Read the model definition and answer for the solid it produces. Units are mm, in the model's axes. Coordinates: 2 decimals unless noted, no trailing zeros. Order: outer loops, then holes, each group sorted by start corner. A loop starts at its lowest first (then second) coordinate and runs counter-clockwise, first axis right, second up. Notation, with made-up numbers: M 30.25,82 L 41.25,82 A24 cw 41.25,105 Z; hole C 83.25,81 d10. An arc over 180 degrees is marked long. Use a Markdown table: item, result. Add a question column.
1) Each of these flat-tipped pins is pushed along its axis until it touches: pin 1 Ø1.3 at (y, z) = (-8.5, -1) entering from -X (3 decimals); pin 2 Ø3.5 at (y, z) = (4, 7.5) entering from -X (3 decimals); pin 3 Ø2 at (y, z) = (-4.76, 8.25) entering from -X. Where does it stop, or does it pass through?
2) Find section A-A on z = 0. Count the separate pieces of the cut face and the enclosed holes in it, plus the area to 3 significant figures.
3) Find section B-B on y = 0. Write down the section's boundary in (x, z) (3 decimals), plus the area to 3 significant figures.
4) Find section C-C on y = 49.5. Write down the section's boundary in (x, z) (3 decimals), plus the area to 3 significant figures.
5) Find the intervals of material crossed by probe 1 along Y at (x, z) = (-0.5, 0) (3 decimals); probe 2 along Y at (x, z) = (-1.25, 0) (3 decimals); probe 3 along Z at (x, y) = (1, -31) (3 decimals), in increasing order. Write a range as [from, to].
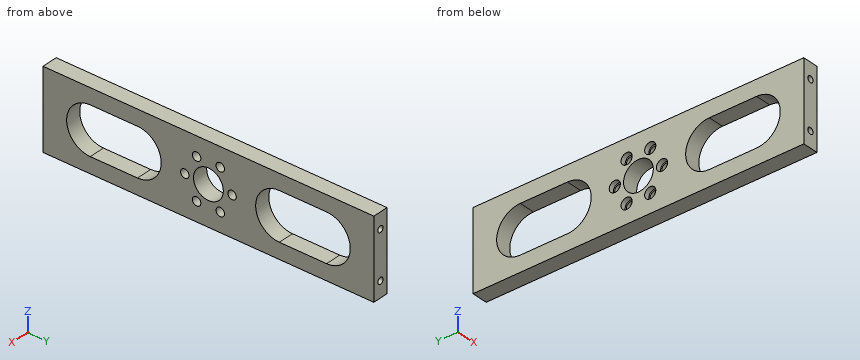
from build123d import *

# Parameters (mm, degrees)
SKETCH1_W                      = 31.75
SKETCH1_H                      = 133.35
BOSS_EXTRUDE1_DEPTH            = 3.175
M3X0_5_TAPPED_HOLE1_AT_2_COUNT = 2
M3X0_5_TAPPED_HOLE1_AT_2_PITCH = 19.05
F_12_0MM_DOWEL_HOLE1_D         = 12
CBORE_FOR_M3_SHCS1_D           = 3.4
CBORE_FOR_M3_SHCS1_DEPTH       = 11.678536948
CBORE_FOR_M3_SHCS1_CBORE_D     = 4.5
CBORE_FOR_M3_SHCS1_CBORE_DEPTH = 2
CBORE_FOR_M3_SHCS1_TIP         = 1.021463052
CUT_EXTRUDE1_DEPTH             = 69.832359759


with BuildPart() as part:
    # Sketch1 → Boss-Extrude1 (new, symmetric)
    with BuildSketch(Plane(origin=(0, 0, 0), x_dir=(0, 0, -1), z_dir=(1, 0, 0))):
        Rectangle(SKETCH1_W, SKETCH1_H)
    extrude(amount=BOSS_EXTRUDE1_DEPTH, both=True)

    # Sketch5 → M3x0.5 Tapped Hole1 (revolve, cut)
    with BuildSketch(Plane(origin=(0, 66.675, -9.525), x_dir=(0, 0, 1), z_dir=(1, 0, 0))):
        Polygon((0, 0), (0, 13.451075774), (1.25, 12.7), (1.25, 0), align=None)
    m3x0_5_tapped_hole1 = revolve(axis=Axis((0, 73.025, -9.525), (0, -1, 0)), mode=Mode.SUBTRACT)

    # M3x0.5 Tapped Hole1 at 2: M3x0.5 Tapped Hole1 ×2
    with Locations(*[(0, 0, i * M3X0_5_TAPPED_HOLE1_AT_2_PITCH) for i in range(1, M3X0_5_TAPPED_HOLE1_AT_2_COUNT)]):
        add(m3x0_5_tapped_hole1, mode=Mode.SUBTRACT)

    # Mirror1: M3x0.5 Tapped Hole1 across plane
    add(m3x0_5_tapped_hole1.mirror(Plane.ZX), mode=Mode.SUBTRACT)

    # Mirror1 copy 1 sketch → Mirror1 copy 1 (revolve, cut)
    with BuildSketch(Plane(origin=(0, -66.675, 9.525), x_dir=(0, 0, 1), z_dir=(1, 0, 0))):
        Polygon((0, 0), (0, -13.451075774), (1.25, -12.7), (1.25, 0), align=None)
    revolve(axis=Axis((0, -73.025, 9.525), (0, -1, 0)), mode=Mode.SUBTRACT)

    # Ø12.0mm Dowel Hole1 (through all)
    with Locations(Plane.ZY.offset(3.175)):
        with Locations((0, 0)):
            Hole(F_12_0MM_DOWEL_HOLE1_D / 2)

    # CBORE for M3 SHCS1
    with Locations(Plane.ZY.offset(3.175)):
        with Locations((8.248891971, -4.7625), (8.248891971, 4.7625), (0, 9.525), (-8.248891971, 4.7625), (-8.248891971, -4.7625), (0, -9.525)):
            CounterBoreHole(CBORE_FOR_M3_SHCS1_D / 2, CBORE_FOR_M3_SHCS1_CBORE_D / 2, CBORE_FOR_M3_SHCS1_CBORE_DEPTH, depth=CBORE_FOR_M3_SHCS1_DEPTH)
            with Locations((0, 0, -(CBORE_FOR_M3_SHCS1_DEPTH + CBORE_FOR_M3_SHCS1_TIP / 2))):  # 118° drill point
                Cone(0, CBORE_FOR_M3_SHCS1_D / 2, CBORE_FOR_M3_SHCS1_TIP, mode=Mode.SUBTRACT)

    # Sketch12 → Cut-Extrude1 (cut, through all)
    with BuildSketch(Plane(origin=(3.175, 0, 0), x_dir=(0, 0, -1), z_dir=(1, 0, 0))):
        with BuildLine():
            Line((-9.525, -28.575), (-9.525, -47.625))
            ThreePointArc((-9.525, -47.625), (0, -57.15), (9.525, -47.625))
            Line((9.525, -47.625), (9.525, -28.575))
            ThreePointArc((9.525, -28.575), (0, -19.05), (-9.525, -28.575))
        make_face()
        with BuildLine():
            Line((9.525, 47.625), (9.525, 28.575))
            ThreePointArc((9.525, 28.575), (0, 19.05), (-9.525, 28.575))
            Line((-9.525, 28.575), (-9.525, 47.625))
            ThreePointArc((-9.525, 47.625), (0, 57.15), (9.525, 47.625))
        make_face()
    extrude(amount=-CUT_EXTRUDE1_DEPTH, mode=Mode.SUBTRACT)


solid = part.part
Check result:
| question | item | result |
|---|---|---|
| 1 | pin 1 | stops at x = -1.175 |
| 1 | pin 2 | stops at x = -3.175 |
| 1 | pin 3 | passes through |
| 2 | separate pieces | 6 |
| 2 | enclosed holes | 0 |
| 2 | area | 239 mm2 |
| 3 | outline | M -3.175,-15.875 L 3.175,-15.875 L 3.175,-6 L -3.175,-6 Z; M -3.175,6 L 3.175,6 L 3.175,15.875 L -3.175,15.875 Z |
| 3 | area | 125 mm2 |
| 4 | outline | M -3.175,-15.875 L 3.175,-15.875 L 3.175,-9.339 L -3.175,-9.339 Z; M -3.175,9.339 L 3.175,9.339 L 3.175,15.875 L -3.175,15.875 Z |
| 4 | area | 83.0 mm2 |
| 5 | probe 1 | y = [-66.675, -57.15], [-19.05, -11.225], [-7.825, -6], [6, 7.825], [11.225, 19.05], [57.15, 66.675] |
| 5 | probe 2 | y = [-66.675, -57.15], [-19.05, -11.775], [-7.275, -6], [6, 7.275], [11.775, 19.05], [57.15, 66.675] |
| 5 | probe 3 | z = [-15.875, -9.525], [9.525, 15.875] |
